from build123d import *

# Parameters (mm, degrees)
SKIZZE1_R                                            = 62
LINEAR_AUSTRAGEN1_DEPTH                              = 25
STIRNSENKUNG_F_R_M6_ZYLINDERSCHRAUBE_MIT_D           = 6.6
STIRNSENKUNG_F_R_M6_ZYLINDERSCHRAUBE_MIT_CBORE_D     = 11
STIRNSENKUNG_F_R_M6_ZYLINDERSCHRAUBE_MIT_CBORE_DEPTH = 9.4
F_12_0_12_DURCHMESSER_BOHRUNG1_REACH                 = 142.872
F_12_0_12_DURCHMESSER_BOHRUNG1_BORE_R                = 5
SKIZZE10_R                                           = 5
SCHNITT_LINEAR_AUSTRAGEN3_DEPTH                      = 0.1
M8_GEWINDEBOHRUNG3_REACH                             = 142.784
M8_GEWINDEBOHRUNG3_BORE_R                            = 3.4


with BuildPart() as part:
    # Skizze1 → Linear austragen1 (new, symmetric)
    with BuildSketch(Plane.XY):
        Circle(SKIZZE1_R)
    extrude(amount=LINEAR_AUSTRAGEN1_DEPTH, both=True)

    # Skizze2 → Schnitt-Rotation1 (revolve, cut)
    with BuildSketch(Plane(origin=(0, 0, 0), x_dir=(0, 0, -1), z_dir=(1, 0, 0)), mode=Mode.PRIVATE) as schnitt_rotation1_sk:
        Polygon((25, 55.05), (13.5, 55.05), (13.5, 45), (-6.4, 45), (-6.4, 40.05), (-17.4, 40.05), (-17.4, 43.55), (-22, 43.55), (-22, 40.05), (-25, 40.05), (-25, 0), (25, 0), align=None)
    revolve(schnitt_rotation1_sk.sketch.rotate(Axis((0, 0, 0), (0, 0, -1)), 90), axis=Axis((0, 0, 0), (0, 0, -1)), mode=Mode.SUBTRACT)

    # Stirnsenkung für M6 Zylinderschraube mit Innensechskant1 (through all)
    with Locations(Plane(origin=(-59.191094396, 8.680738145, 25), x_dir=(1, 0, 0), z_dir=(0, 0, 1))):
        with Locations((59.191094396, 41.319261855), (102.492364585, -33.680738145), (15.889824207, -33.680738145)):
            CounterBoreHole(STIRNSENKUNG_F_R_M6_ZYLINDERSCHRAUBE_MIT_D / 2, STIRNSENKUNG_F_R_M6_ZYLINDERSCHRAUBE_MIT_CBORE_D / 2, STIRNSENKUNG_F_R_M6_ZYLINDERSCHRAUBE_MIT_CBORE_DEPTH)

    # Ø12.0 (12) Durchmesser Bohrung1 bore → Ø12.0 (12) Durchmesser Bohrung1 (cut, up to next)
    with BuildSketch(Plane(origin=(-62, 0, 0), x_dir=(0, 1, 0), z_dir=(-1, 0, 0)), mode=Mode.PRIVATE) as f_12_0_12_durchmesser_bohrung1_sk1:
        with Locations((0, 5)):
            Circle(F_12_0_12_DURCHMESSER_BOHRUNG1_BORE_R)
    f_12_0_12_durchmesser_bohrung1_tool1 = extrude(f_12_0_12_durchmesser_bohrung1_sk1.sketch, amount=-F_12_0_12_DURCHMESSER_BOHRUNG1_REACH, mode=Mode.PRIVATE) & part.part
    f_12_0_12_durchmesser_bohrung1 = f_12_0_12_durchmesser_bohrung1_tool1.solids().sort_by_distance((-62, 0, -5))[0]
    add(f_12_0_12_durchmesser_bohrung1, mode=Mode.SUBTRACT)

    # Spiegeln1: Ø12.0 (12) Durchmesser Bohrung1 across plane
    add(f_12_0_12_durchmesser_bohrung1.mirror(Plane(origin=(0, 0, 0), x_dir=(0, 0, 1), z_dir=(1, 0, 0))), mode=Mode.SUBTRACT)

    # Skizze10 → Schnitt-Linear austragen3 (cut)
    with BuildSketch(Plane(origin=(0, -62, 0), x_dir=(1, 0, 0), z_dir=(0, 1, 0))):
        Circle(SKIZZE10_R)
    extrude(amount=SCHNITT_LINEAR_AUSTRAGEN3_DEPTH, mode=Mode.SUBTRACT)

    # M8 Gewindebohrung3 bore → M8 Gewindebohrung3 (cut, up to next)
    with BuildSketch(Plane(origin=(0, -61.9, 0), x_dir=(-1, 0, 0), z_dir=(0, -1, 0)), mode=Mode.PRIVATE) as m8_gewindebohrung3_sk1:
        Circle(M8_GEWINDEBOHRUNG3_BORE_R)
    m8_gewindebohrung3_tool1 = extrude(m8_gewindebohrung3_sk1.sketch, amount=-M8_GEWINDEBOHRUNG3_REACH, mode=Mode.PRIVATE) & part.part
    add(m8_gewindebohrung3_tool1.solids().sort_by_distance((0, -61.9, 0))[0], mode=Mode.SUBTRACT)


solid = part.part
The listing builds one solid part. Answer for the finished solid, in the listing's coordinates (mm). A direction names the side the tool comes from. Coordinates: 2 decimals unless noted, no trailing zeros. Write each loop counter-clockwise with the first axis right and the second up, starting at its lowest first coordinate (ties: lowest second). Pieces come first, ordered by that corner, then holes. Notation, with made-up numbers: M 62,14.25 L 92,14.25 A21 cw 92,35.25 Z; hole C 86.5,-3.5 d3. An arc over 180 degrees is marked long. Use one line per item in the form item = value.
Item 1: For faces 1 (the face through (39.25, -21.28, 20.37)), 2 (the face through (0.74, -53.5, 3.32)), 3 (the face through (39, 13, 22)), 4 (the face through (40.25, -26.26, 0.85)), 5 (the face through (-11.93, 53.74, -19.17)), determine the directions among +Z, -Z, +X, -X, +Y, -Y from which every point of the face is accessible in a straight line to the end or side of a thin tool.
Model answer:
face_1 = +Z
face_2 = -Y
face_3 = none
face_4 = +Z, -Z
face_5 = -Z
Item 2: The mould has two halves that part along Z. Classify faces 6 (the face through (-53.48, -1.08, -0.12)), 7 (the face through (40.5, 0.9, 25)), 8 (the face through (-38.055, -23.348, 20.366)): released by +Z, released by -Z, zero draft, split by the parting line, or undercut.
Model answer:
face_6 = undercut
face_7 = released by +Z
face_8 = zero draft
Item 3: Find section B-B, the plane z = -8. Give the vertices of the cut face in (x, y), plus the area to 3 significant figures.
Model answer:
outline = M -61.87,-4 A62 ccw 61.87,-4 L 44.82,-4 A45 cw -44.82,-4 Z; M -61.87,4 L -44.82,4 A45 cw 44.82,4 L 61.87,4 A62 ccw Z; hole C -43.3,-25 d6.6; hole C 0,50 d6.6; hole C 43.3,-25 d6.6
area = 5,340 mm2
Item 4: Find section C-C, the plane x = 10. Give the vertices of the cut face in (y, z).
Model answer:
outline = M -61.19,-25 L -54.13,-25 L -54.13,-13.5 L -43.87,-13.5 L -43.87,6.4 L -38.78,6.4 L -38.78,17.4 L -42.39,17.4 L -42.39,22 L -38.78,22 L -38.78,25 L -61.19,25 Z; M 38.78,6.4 L 43.87,6.4 L 43.87,-13.5 L 54.13,-13.5 L 54.13,-25 L 61.19,-25 L 61.19,25 L 38.78,25 L 38.78,22 L 42.39,22 L 42.39,17.4 L 38.78,17.4 Z
Item 5: Given P1, Ø10, axis at y = -1, z = 18, coming from the +X side; P2, Ø10, axis at x = 43.3, y = -25, coming from the -Z side; P3, Ø8, axis at x = -43.5, z = -3.5, coming from the +Y side; P4, Ø4, axis at x = -45, z = -2, coming from the -Y side, each flat-ended and moving along its own axis, determine where each tip first touches the part or whether it passes through.
Model answer:
P1 = 62
P2 = -13.5
P3 = 47.79
P4 = -44.67
Item 6: Find the intervals of material crossed by probe 1 along Y at (x, z) = (0, -6.5); probe 2 along Z at (x, y) = (32.5, -41.5); probe 3 along X at (y, z) = (-31.5, 7), in increasing order.
Model answer:
probe_1 = -62 to -45, 45 to 46.7, 53.3 to 62
probe_2 = -13.5 to 25
probe_3 = -53.4 to -24.73, 24.73 to 53.4
Item 7: Find section A-A, the plane y = 0. Give the number of separate pieces and of enclosed holes in the cut face, plus the area to 3 significant figures.
Model answer:
separate_pieces = 4
enclosed_holes = 0
area = 1,280 mm2
Item 8: Find section D-D, the plane z = 12. Give the vertices of the cut face in (x, y).
Model answer:
outline = C 0,0 d124; hole C -43.3,-25 d6.6; hole C 0,0 d80.1; hole C 0,50 d6.6; hole C 43.3,-25 d6.6
